Autodesk Inventor part; units mm, degrees
ref_plane "YZ Plane" through (0, 0, 0) normal (1, 0, 0) x (0, 1, 0)
ref_plane "XZ Plane" through (0, 0, 0) normal (0, 1, 0) x (-1, 0, 0)
ref_plane "XY Plane" through (0, 0, 0) normal (0, 0, 1) x (1, 0, 0)
sketch "Sketch1" plane through (0, 0, 0) normal (0, 1, 0) x (-1, 0, 0)
  line L0 (0, 0) -> (0, -10)
  line L1 (0, -10) -> (10, -10)
  line L2 (10, -10) -> (0, 0)
  line L3 (0, -10) -> (-10, -10)
  line L4 (-10, -10) -> (0, 0)
  line L5 (0, 0) -> (17.6777, -17.6777)
  line L6 (0, 0) -> (-17.6777, -17.6777)
  line L7 (-17.6777, -17.6777) -> (17.6777, -17.6777)
  line L8 (0, -17.6777) -> (0, -29.9777)
  circle A0 centre (0, -29.9777) radius 9.65
  circle A1 centre (0, -29.9777) radius 6
  line L9 (17.6777, -17.6777) -> (22.6777, -17.6777)
  line L10 (-17.6777, -17.6777) -> (-22.6777, -17.6777)
  line L11 (-22.6777, -17.6777) -> (-22.6777, -42.6777)
  line L12 (-22.6777, -42.6777) -> (22.6777, -42.6777)
  line L13 (22.6777, -42.6777) -> (22.6777, -17.6777)
  dimension "d0" = 10
  dimension "d1" = 10
  dimension "d2" = 10
  dimension "d3" = 25
  dimension "d4" = 25
  dimension "d5" = 12.3
  dimension "d6" = 19.3
  dimension "d7" = 12
  dimension "d8" = 5
  dimension "d9" = 5
  dimension "d10" = 25
extrude "Extrusion1" add sketch "Sketch1" along normal blind 3 contours A0
extrude "Extrusion2" add sketch "Sketch1" along normal blind 9 contours L9 L13 L12 L11 L10 L7
sketch "Sketch2" plane through (-22.6777, 0, -17.6777) normal (0, 0, 1) x (1, 0, 0)
  line L0 (0, 0) -> (0, 9)
  line L1 (0, 4.5) -> (5, 4.5)
  line L2 (45.3553, 9) -> (45.3553, 0)
  line L3 (45.3553, 4.5) -> (40.3553, 4.5)
  circle A0 centre (5, 4.5) radius 2.6
  circle A1 centre (40.3553, 4.5) radius 2.6
  point P0 (22.6777, 0)
  dimension "d15" = 5
  dimension "d16" = 5
  dimension "d17" = 5.2
  dimension "d18" = 5.2
extrude "Extrusion3" cut sketch "Sketch2" against normal blind 26
fillet "Fillet1" radius 4 2 edges at (22.6777, 4.5, -42.6777) (-22.6777, 4.5, -42.6777)
properties part number "bearing_holder_corner_tb"
Geometry: final body of the model. Coordinates: model frame, mm. A direction names the side the tool comes from. Give positions to 0.01 mm unless a question says otherwise; leave off trailing zeros. Write each loop counter-clockwise with the first axis right and the second up, starting at its lowest first coordinate (ties: lowest second). Pieces come first, ordered by that corner, then holes. Notation, with made-up numbers: (16.5, 85) - (70.5, 85) arc R8 ccw to (70.5, 95) - close; hole circle Ø4 at (-20, 28.25). An arc over 180 degrees is marked (long way). Return JSON: item names as keys, results as strings. Group by question number.
1) Section A-A on z = -27.25. Return the cut outline in (x, y).
2) First-contact query: P1, Ø8, axis at x = -2.5, z = -29.5, coming from the +Y side. Flat tip, straight axial feed; report the tip coordinate or a pass-through.
3) Line query: line 1 (X direction, y = 4.5, z = -41.5); line 2 (X direction, y = 6.25, z = -28.75); line 3 (X direction, y = 2.75, z = -20.5). Output: solid intervals per line, ascending.
4) Section C-C on x = 0. Return the cut outline in (y, z).
5) Mould query, pull axis Y, two halves, no side actions, for faces 1 (the flat face through (5, 0, -24)), 2 (the flat face through (0, 4, -42.678)), 3 (the cylindrical face through (-20.275, 4.614, -30.003)), 4 (the cylindrical face through (20.158, 5.281, -30.003)). Classes: released by +Y, released by -Y, zero draft, split by the parting line, or undercut.
6) Section B-B on y = 5.25. Return the cut outline in (x, z), plus the area to 3 significant figures.
7) Section D-D on z = -23. Return the cut outline in (x, y).
8) Set-up query: faces 5 (the flat face through (22.678, 4, -28)), 6 (the flat face through (-6.3, 3, -29.8)). Return all of +Z, -Z, +X, -X, +Y, -Y with unobstructed straight access to the full face (end or side cutting, diameter ignored); none if empty.
Filled in:
{
 "1": {"outline": "(-22.68, 0) - (-5.34, 0) - (-5.34, 3) - (-9.26, 3) - (-9.26, 9) - (-22.68, 9) - close; (5.34, 0) - (22.68, 0) - (22.68, 9) - (9.26, 9) - (9.26, 3) - (5.34, 3) - close; hole circle Ø5.2 at (-17.68, 4.5); hole circle Ø5.2 at (17.68, 4.5)"},
 "2": {"P1": "stops at y = 3"},
 "3": {"line 1": "x = -21.51 to -20.28, -15.08 to 15.08, 20.28 to 21.51", "line 2": "x = -22.68 to -19.6, -15.75 to -9.57, 9.57 to 15.75, 19.6 to 22.68", "line 3": "x = -22.68 to -19.6, -15.75 to 15.75, 19.6 to 22.68"},
 "4": {"outline": "(0, -42.68) - (9, -42.68) - (9, -39.63) - (3, -39.63) - (3, -35.98) - (0, -35.98) - close; (0, -23.98) - (3, -23.98) - (3, -20.33) - (9, -20.33) - (9, -17.68) - (0, -17.68) - close"},
 "5": {"face 1": "released by -Y", "face 2": "zero draft", "face 3": "undercut", "face 4": "undercut"},
 "6": {"outline": "(-22.68, -38.68) arc R4 ccw to (-20.17, -42.39) - (-20.17, -17.68) - (-22.68, -17.68) - close; (-15.19, -42.68) - (15.19, -42.68) - (15.19, -17.68) - (-15.19, -17.68) - close; (20.17, -42.39) arc R4 ccw to (22.68, -38.68) - (22.68, -17.68) - (20.17, -17.68) - close; hole circle Ø19.3 at (0, -29.98)", "area": "586 mm^2"},
 "7": {"outline": "(-22.68, 0) - (22.68, 0) - (22.68, 9) - (6.67, 9) - (6.67, 3) - (-6.67, 3) - (-6.67, 9) - (-22.68, 9) - close; hole circle Ø5.2 at (-17.68, 4.5); hole circle Ø5.2 at (17.68, 4.5)"},
 "8": {"face 5": "+Z, -Z, +X, +Y, -Y", "face 6": "+Y"}
}
